from build123d import *

# Parameters (mm, degrees)
SKETCH1_R           = 1
BOSS_EXTRUDE1_DEPTH = 2
SKETCH3_R           = 2
SKETCH3_R_2         = 1
BOSS_EXTRUDE3_DEPTH = 6


with BuildPart() as part:
    # Sketch1 → Boss-Extrude1 (new body)
    with BuildSketch(Plane(origin=(0, 0, 0), x_dir=(1, 0, 0), z_dir=(0, 1, 0))):
        with BuildLine():
            Line((10.165797332, 16.468729903), (-1.584202668, 1.220779221))
            ThreePointArc((-1.584202668, 1.220779221), (-2, 0), (-1.584202668, -1.220779221))
            Line((-1.584202668, -1.220779221), (10.165797332, -16.468729903))
            ThreePointArc((10.165797332, -16.468729903), (12.970779221, -16.83215335), (13.334202668, -14.027171461))
            Line((13.334202668, -14.027171461), (2.524929468, 0))
            Line((2.524929468, 0), (13.334202668, 14.027171461))
            ThreePointArc((13.334202668, 14.027171461), (12.970779221, 16.83215335), (10.165797332, 16.468729903))
        make_face()
        with Locations(Location((0, 0, 0), (0, 0, 270))):
            Circle(SKETCH1_R, mode=Mode.SUBTRACT)
        with Locations(Location((11.75, 15.247950682, 0), (0, 0, 270))):
            Circle(SKETCH1_R, mode=Mode.SUBTRACT)
        with Locations(Location((11.75, -15.247950682, 0), (0, 0, 90))):
            Circle(SKETCH1_R, mode=Mode.SUBTRACT)
    extrude(amount=BOSS_EXTRUDE1_DEPTH)

    # Sketch3 → Boss-Extrude3 (add)
    # profile 1 of 2: a face of its own
    with BuildSketch(Plane(origin=(0, 2, 0), x_dir=(1, 0, 0), z_dir=(0, 1, 0))):
        with Locations(Location((11.75, 15.247950682, 0), (0, 0, 142.382320334))):
            Circle(SKETCH3_R)
        with Locations(Location((11.75, 15.247950682, 0), (0, 0, 270))):
            Circle(SKETCH3_R_2, mode=Mode.SUBTRACT)
    # profile 2 of 2: a face of its own
    with BuildSketch(Plane(origin=(0, 2, 0), x_dir=(1, 0, 0), z_dir=(0, 1, 0))):
        with Locations(Location((11.75, -15.247950682, 0), (0, 0, 37.617679666))):
            Circle(SKETCH3_R)
        with Locations(Location((11.75, -15.247950682, 0), (0, 0, 90))):
            Circle(SKETCH3_R_2, mode=Mode.SUBTRACT)
    extrude(amount=BOSS_EXTRUDE3_DEPTH)


solid = part.part
CAD build for the part. Positions are in the model's coordinates, mm. A direction names the side the tool comes from. Round coordinates to 2 decimals unless told otherwise and drop trailing zeros. Write each loop counter-clockwise with the first axis right and the second up, starting at its lowest first coordinate (ties: lowest second). Pieces come first, ordered by that corner, then holes. Notation, with made-up numbers: M 47,-7.5 L 56,-7.5 A22 ccw 56,8.5 Z; hole C -36.5,78 d2. An arc over 180 degrees is marked long. Use a Markdown table: item, result. Add a question column.
1. Flat gauge pins, fed straight in: P1, Ø1, axis at x = 8, y = 7, coming from the -Z side; P2, Ø1.5, axis at x = 9.5, y = 3, coming from the +Z side; P3, Ø2, axis at x = 9.5, y = 4.5, coming from the +Z side; P4, Ø4, axis at x = 8, y = 5, coming from the -Z side. Where does each tip first touch, or does it go through?
2. Slice it at C-C on x = 0. Give the cut face in (y, z).
3. Slice it at B-B on z = 0.5. Give the cut face in (x, y).
4. 3-axis set-ups, long thin cutter, end or side, ignore diameter. For faces 5 (the face through (13.285, 3.944, -16.53)), 6 (the face through (8.005, 0.986, 7.112)), 7 (the face through (4.21, 0.99, 8.74)): which of +Z, -Z, +X, -X, +Y, -Y reach the whole face in a straight line?
5. Pull direction Z, two halves, no side cores. Call faces 1 (the face through (-1, 1, 0)), 2 (the face through (12, 8, 14)), 3 (the face through (11.367, 3.944, -14.324)), 4 (the face through (4.37, 0.99, -8.95)): released by +Z, released by -Z, zero draft, split by the parting line, or undercut.
6. Drill centre lines: probe 1 along Z at (x, y) = (12, 3); probe 2 along Y at (x, z) = (7.75, 13); probe 3 along X at (y, z) = (5, 15). Where is each one in solid material? Low to high.
7. Slice it at A-A on y = 3.75. Give the cut face in (x, z).
Reply:
| question | item | result |
|---|---|---|
| 1 | P1 | passes through |
| 1 | P2 | stops at z = 16.57 |
| 1 | P3 | stops at z = 16.81 |
| 1 | P4 | stops at z = -16.22 |
| 2 | outline | M 0,-3.28 L 2,-3.28 L 2,-1 L 0,-1 Z; M 0,1 L 2,1 L 2,3.28 L 0,3.28 Z |
| 3 | outline | M -1.94,0 L -0.87,0 L -0.87,2 L -1.94,2 Z; M 0.87,0 L 2.91,0 L 2.91,2 L 0.87,2 Z |
| 4 | face 5 | +Y |
| 4 | face 6 | +X, +Y, -Y |
| 4 | face 7 | +Z, -X, +Y, -Y |
| 5 | face 1 | undercut |
| 5 | face 2 | zero draft |
| 5 | face 3 | undercut |
| 5 | face 4 | released by -Z |
| 6 | probe 1 | z = -17.23 to -16.22, -14.28 to -13.26, 13.26 to 14.28, 16.22 to 17.23 |
| 6 | probe 2 | y = 0 to 2 |
| 6 | probe 3 | x = 9.77 to 10.78, 12.72 to 13.73 |
| 7 | outline | C 11.75,-15.25 d4; C 11.75,15.25 d4; hole C 11.75,-15.25 d2; hole C 11.75,15.25 d2 |
